from build123d import *

# Parameters (mm, degrees)
F0_R     = 38.5379103623
F0_R_2   = 16.6938076384
F1_DEPTH = 25.4
F2_R     = 12.69999


# Not quite as in the source:
# - a fillet or chamfer that OpenCascade refuses, or shapes differently, is made with other operations: its cross-section is extruded or revolved along the edge and cut away or added
# - a fillet or chamfer is up to 0.001 mm smaller than in the source, because OpenCascade refuses the exact size


with BuildPart() as f1:
    # F0 (on Top) → F1 (new body)
    with BuildSketch(Plane.XY):
        Circle(F0_R)
        Circle(F0_R_2, mode=Mode.SUBTRACT)
    extrude(amount=F1_DEPTH)

    # F2 (radius 12.7 in the source; OpenCascade refuses exactly that, so slightly less here)
    f2_edges = [f1.edges().sort_by_distance(p)[0] for p in [
        (-38.53791, 0, 25.4),
        (-38.53791, 0, 0),
    ]]
    fillet(f2_edges, radius=F2_R)

    # F3: fillet of radius 12.7 on 2 edges, made by hand

    # F3_s1 → F3_t2 (revolve, cut)
    with BuildSketch(Plane.XZ):
        with BuildLine():
            ThreePointArc((25.8379203623, 25.4), (19.2338428647, 20.8280140909), (16.6938076384, 13.2079671228))
            Line((16.6938076384, 13.2079671228), (16.6938076384, 25.4))
            Line((16.6938076384, 25.4), (25.8379203623, 25.4))
        make_face()
    revolve(axis=Axis((0, 0, 25.4), (0, 0, 1)), mode=Mode.SUBTRACT)

    # F3_s3 → F3_t4 (revolve, cut)
    with BuildSketch(Plane.XZ):
        with BuildLine():
            ThreePointArc((25.8379203623, 0), (19.2338428647, 4.5719859091), (16.6938076384, 12.1920328772))
            Line((16.6938076384, 12.1920328772), (16.6938076384, 0))
            Line((16.6938076384, 0), (25.8379203623, 0))
        make_face()
    revolve(axis=Axis((0, 0, 0), (0, 0, 1)), mode=Mode.SUBTRACT)


solid = f1.part
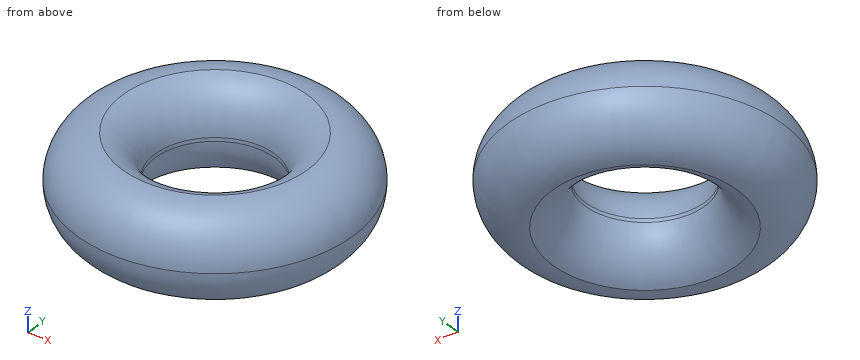
Can you work these out from the model? Positions are in its coordinate system, mm. Coordinates: 2 decimals unless noted, no trailing zeros. Write each loop counter-clockwise with the first axis right and the second up, starting at its lowest first coordinate (ties: lowest second). Pieces come first, ordered by that corner, then holes.
Q1. Please list where these lines run through material, in increasing order: L1, parallel to Y at x = 0, z = 12.65; L2, parallel to X at y = -10, z = 2.75; L3, parallel to Y at x = -9, z = 10.5.
Results found:
L1: y = -38.54 to -16.69, 16.69 to 38.54
L2: x = -32.21 to -18.35, 18.35 to 32.21
L3: y = -37.27 to -14.19, 14.19 to 37.27
Q2. For P1, Ø10, axis at x = 11, z = 12, coming from the -Y side; P2, Ø5, axis at x = 8, z = 21, coming from the +Y side; P3, Ø1, axis at x = 13, y = 28.5, coming from the -Z side, each with a flat end and sliding along its axis, tell me the tip position at first contact or that it passes through.
Results found:
P1: stops at y = -38.06
P2: stops at y = 36.36
P3: stops at z = 1.02
Q3. Imagine slicing it at C-C, the plane z = 18.75. List the corners of the cut face in (x, y) for me.
Results found:
outline: circle Ø74.01 at (0, 0); hole circle Ø35.93 at (0, 0)
Q4. Imagine slicing it at D-D, the plane z = 23. List the corners of the cut face in (x, y) for me, plus the area to 3 significant figures.
Results found:
outline: circle Ø66.54 at (0, 0); hole circle Ø42.61 at (0, 0)
area: 2,050 mm2
